from build123d import *

# Parameters (mm, degrees)
BOSS_EXTRUDE1_DEPTH = 3.175
SKETCH2_R           = 2.5796875
CUT_EXTRUDE1_DEPTH  = 4.175


with BuildPart() as part:
    # Sketch1 → Boss-Extrude1 (new body)
    with BuildSketch(Plane.XY):
        Polygon((-441.3957506, 526.537652812), (193.6042494, 526.537652812), (193.6042494, -83.062347188), (104.7042494, -83.062347188), (104.7042494, 374.137652812), (-352.4957506, 374.137652812), (-352.4957506, -83.062347188), (-441.3957506, -83.062347188), (-441.3957506, 36.485330073), align=None)
    extrude(amount=BOSS_EXTRUDE1_DEPTH)

    # Sketch2 → Cut-Extrude1 (cut, through all)
    with BuildSketch(Plane.XY.offset(3.175)):
        with Locations((-396.9457506, 221.737652812)):
            Circle(SKETCH2_R)
        with Locations((149.1542494, 221.737652812)):
            Circle(SKETCH2_R)
    extrude(amount=-CUT_EXTRUDE1_DEPTH, mode=Mode.SUBTRACT)


solid = part.part
Can you work these out from the model? Positions are in its coordinate system, mm. Coordinates: 2 decimals unless noted, no trailing zeros. Order: outer loops, then holes, each group sorted by start corner. A loop starts at its lowest first (then second) coordinate and runs counter-clockwise, first axis right, second up. Notation, with made-up numbers: (42.25, 77) - (81.25, 77) arc R20 cw to (81.25, 110) - close; hole circle Ø9 at (19.25, 26). An arc over 180 degrees is marked (long way). Answer as a JSON object with one key per item and string values. Group by question number.
Q1. Imagine slicing it at C-C (x = -36.5). Please give me the cut outline in (y, z) (3 decimals), and give its area (3 significant figures).
Q2. Imagine slicing it at A-A (y = 136.5). Please give me the cut outline in (x, z) (3 decimals).
Q3. Imagine slicing it at B-B (z = 2.4). Please give me the cut outline in (x, y).
Q4. I need wall thicknesses on line 1 (X direction, y = -45.5, z = 1.3); line 2 (Y direction, x = 15.5, z = 1.75). Which ranges of each line are inside material? Lowest first, please. Write a range as from..to.
Q5. Will this pin go through, and if not, where does the flat tip stop? P1, Ø1.5, axis at x = -19, z = 2.5, coming from the -Y side.
Determined:
{
 "1": {"outline": "(374.138, 0) - (526.538, 0) - (526.538, 3.175) - (374.138, 3.175) - close", "area": "484 mm2"},
 "2": {"outline": "(-441.396, 0) - (-352.496, 0) - (-352.496, 3.175) - (-441.396, 3.175) - close; (104.704, 0) - (193.604, 0) - (193.604, 3.175) - (104.704, 3.175) - close"},
 "3": {"outline": "(-441.4, -83.06) - (-352.5, -83.06) - (-352.5, 374.14) - (104.7, 374.14) - (104.7, -83.06) - (193.6, -83.06) - (193.6, 526.54) - (-441.4, 526.54) - close; hole circle Ø5.16 at (-396.95, 221.74); hole circle Ø5.16 at (149.15, 221.74)"},
 "4": {"line 1": "x = -441.4..-352.5, 104.7..193.6", "line 2": "y = 374.14..526.54"},
 "5": {"P1": "stops at y = 374.14"}
}
